Can you work these out from the model? Positions are in its coordinate system, mm. A direction names the side the tool comes from. Coordinates: 2 decimals unless noted, no trailing zeros. Order: outer loops, then holes, each group sorted by start corner. A loop starts at its lowest first (then second) coordinate and runs counter-clockwise, first axis right, second up. Notation, with made-up numbers: (49.5, 35) -> (80.5, 35) arc R27 ccw to (80.5, 57) -> close; hole circle Ø5 at (63.5, 22). An arc over 180 degrees is marked (long way). Return JSON: item names as keys, results as strings. Group by question number.
1) Thinking about a two-plate mould opening in X: for faces 1 (the cylindrical face through (61.508, 43.655, 10.14)), 2 (the flat face through (55.58, 44.5, 10.14)), 3 (the cylindrical face through (73.374, 38.23, 9.86)), which applies, +X half, -X half, draft (parallel to the pull), parting line (faces both ways), or undercut?
2) For faces 4 (the cylindrical face through (67.82, 40.29, 10.14)), 5 (the flat face through (67.575, 43.34, 10.14)), 6 (the flat face through (64.227, 45.075, 10.14)), which set-ups out of +Z, -Z, +X, -X, +Y, -Y let a thin tool reach every point of the face, with its end or its side?
3) For pin 1 (4 mm diameter, centred on x = 28.5, z = 7, fed in from +Y); pin 2 (1 mm diameter, centred on x = 46.5, y = 39.5, fed in from +Z); pin 3 (10 mm diameter, centred on y = 36.5, z = 12, fed in from -X); pin 4 (8 mm diameter, centred on y = 1, z = 11, fed in from -X), each with a flat end and sliding along its axis, tell me the tip position at first contact or that it passes through.
4) If we section it at D-D, the plane y = -4.5: Please give me the cut outline in (x, z), then the cut area to 3 significant figures.
5) If we section it at A-A, the plane y = 27.5: Please give me the cut outline in (x, z), then the cut area to 3 significant figures.
6) If we section it at C-C, the plane x = 30: Please give me the cut outline in (y, z).
7) If I drill on probe 1 along X at (y, z) = (40, 11); probe 2 along X at (y, z) = (34, 10.75); probe 3 along Y at (x, z) = (49, 16.25), over which ranges is the centre line in solid material (lowest first)? Write a range as from..to.
from build123d import *

# Parameters (mm, degrees)
SKETCH1_R           = 13.348229866
SKETCH1_R_2         = 2
BOSS_EXTRUDE1_DEPTH = 20
CUT_EXTRUDE4_DEPTH  = 91.243420293
CIRPATTERN7_COUNT   = 4
CIRPATTERN7_ANGLE   = 135
CIRPATTERN9_DEPTH   = 20


# Read off the part's stored shape, not the designer's step: CirPattern9
with BuildPart() as part:
    # Sketch1 → Boss-Extrude1 (new body)
    # profile 1 of 2: a face of its own
    with BuildSketch(Plane.XY):
        with Locations((-60.602362619, 34.350667158)):
            Circle(SKETCH1_R)
        with Locations((-60.602362619, 34.350667158)):
            Circle(SKETCH1_R_2, mode=Mode.SUBTRACT)
    # profile 2 of 2: a face of its own
    with BuildSketch(Plane.XY):
        with BuildLine():
            Line((-66.137497339, 22.204164608), (-31.323181793, -12.610150938))
            Line((-31.323181793, -12.610150938), (-17.655141573, 1.057889282))
            Line((-17.655141573, 1.057889282), (-47.664311726, 31.067059435))
            ThreePointArc((-47.664311726, 31.067059435), (-54.828410927, 22.315854221), (-66.137497339, 22.204164608))
        make_face()
    extrude(amount=BOSS_EXTRUDE1_DEPTH)

    # Sketch2 → Cut-Extrude4 (cut, symmetric)
    with BuildSketch(Plane.XY):
        with BuildLine():
            Line((-169.23850632, 174.404401772), (-68.783555417, 44.897862281))
            Line((-68.783555417, 44.897862281), (-66.331936624, 41.737234923))
            ThreePointArc((-66.331936624, 41.737234923), (-67.840347325, 40.266829683), (-68.981232991, 38.496017917))
            Line((-68.981232991, 38.496017917), (-72.566455217, 40.269765811))
            Line((-72.566455217, 40.269765811), (-219.470747071, 112.948992325))
            Line((-219.470747071, 112.948992325), (-473.273699138, 320.401698382))
            Line((-473.273699138, 320.401698382), (-423.041458386, 381.857107829))
            Line((-423.041458386, 381.857107829), (-169.23850632, 174.404401772))
        make_face()
    cut_extrude4 = extrude(amount=CUT_EXTRUDE4_DEPTH, both=True, mode=Mode.SUBTRACT)

    # CirPattern7: Cut-Extrude4 ×4 about axis
    cirpattern7_axis = Axis((-60.602362619, 34.350667158, 20), (0, 0, -1))
    for i in range(1, CIRPATTERN7_COUNT):
        add(cut_extrude4.rotate(cirpattern7_axis, i * CIRPATTERN7_ANGLE / (CIRPATTERN7_COUNT - 1)), mode=Mode.SUBTRACT)

    # CirPattern9 outline → CirPattern9 (cut)
    with BuildSketch(Plane.XY):
        with BuildLine():
            Line((-73.247688421, 30.076210947), (-69.45832431, 31.357116731))
            ThreePointArc((-69.45832431, 31.357116731), (-69.903749327, 33.41599773), (-69.876875408, 35.522338682))
            Line((-69.876875408, 35.522338682), (-73.845332718, 36.023683446))
            ThreePointArc((-73.845332718, 36.023683446), (-73.883705678, 33.016063436), (-73.247688421, 30.076210947))
        make_face()
        with BuildLine():
            Line((-67.988930384, 28.621093153), (-71.149557741, 26.16947436))
            ThreePointArc((-71.149557741, 26.16947436), (-69.049983017, 24.015632075), (-66.521461271, 22.386574559))
            Line((-66.521461271, 22.386574559), (-64.747713378, 25.971796785))
            ThreePointArc((-64.747713378, 25.971796785), (-66.518525144, 27.112682451), (-67.988930384, 28.621093153))
        make_face()
    extrude(amount=CIRPATTERN9_DEPTH, mode=Mode.SUBTRACT)


with BuildPart() as body_2:
    # Mirror2: mirrored copy
    add(part.part.mirror(Plane(origin=(0, 0, 0), x_dir=(0, 0, 1), z_dir=(1, 0, 0))))


solid = body_2.part
Result sheet:
{
 "1": {"face 1": "undercut", "face 2": "-X half", "face 3": "+X half"},
 "2": {"face 4": "+Z, -Z", "face 5": "+Z, -Z, +X", "face 6": "+Z, -Z, +Y"},
 "3": {"pin 1": "stops at y = 13.9", "pin 2": "passes through", "pin 3": "stops at x = 47.36", "pin 4": "stops at x = 17.66"},
 "4": {"outline": "(23.21, 0) -> (39.43, 0) -> (39.43, 20) -> (23.21, 20) -> close", "area": "324 mm2"},
 "5": {"outline": "(44.1, 0) -> (66.96, 0) -> (66.96, 20) -> (44.1, 20) -> close; (69.43, 0) -> (72.06, 0) -> (72.06, 20) -> (69.43, 20) -> close", "area": "510 mm2"},
 "6": {"outline": "(-11.29, 0) -> (13.4, 0) -> (13.4, 20) -> (-11.29, 20) -> close"},
 "7": {"probe 1": "x = 48.51..68.05, 72.02..72.7", "probe 2": "x = 51.26..58.63, 62.57..69.94", "probe 3": "y = 5.07..32.88, 38.27..40.95"}
}
